The figure shows three views and two pictorial views of one solid part (mm, origin at its lowest corner). Answer the questions. A direction names the side the tool comes from. Coordinates: 2 decimals unless noted, no trailing zeros. Loops run counter-clockwise (first coordinate to the right, second up) from the corner with the lowest first, then second, coordinate; pieces in that order, holes last. Notation, with made-up numbers: M 85,-1 L 101,-1 A30 ccw 101,28 Z; hole C 82.5,75.25 d1. An arc over 180 degrees is marked long. Answer as a JSON object with one key per item and string values. Group by question number.
1. Straight lines are drawn through the part: L1, parallel to Y at x = 2.75, z = 2.25; L2, parallel to Z at x = 4, y = 11; L3, parallel to X at y = 5.5, z = 3. For each, find the intervals that lie inside material, in ascending order.
2. A cutting plane is placed at C-C on y = 12.75. Give the vertices of the cut face in (x, z).
3. Given pin 1 (0.5 mm diameter, centred on x = 3.5, y = 15, fed in from +Z); pin 2 (2 mm diameter, centred on x = 3, z = 3.5, fed in from +Y); pin 3 (3 mm diameter, centred on x = 2.5, y = 14, fed in from +Z); pin 4 (1.5 mm diameter, centred on y = 9.5, z = 3.5, fed in from -X), each flat-ended and moving along its own axis, determine where each tip first touches the part or whether it passes through.
4. A cutting plane is placed at A-A on y = 15.25. Give the vertices of the cut face in (x, z) (1 decimal).
5. For the marked faces 4, 5 and 6, determine the directions among +Z, -Z, +X, -X, +Y, -Y from which every point of the face is accessible in a straight line to the end or side of a thin tool.
6. A cutting plane is placed at B-B on x = 3.1. Give the vertices of the cut face in (y, z).
7. Determine the mould class of the marked faces 1, 2 and 3 for opening direction Z: released by +Z, released by -Z, zero draft, split by the parting line, or undercut.
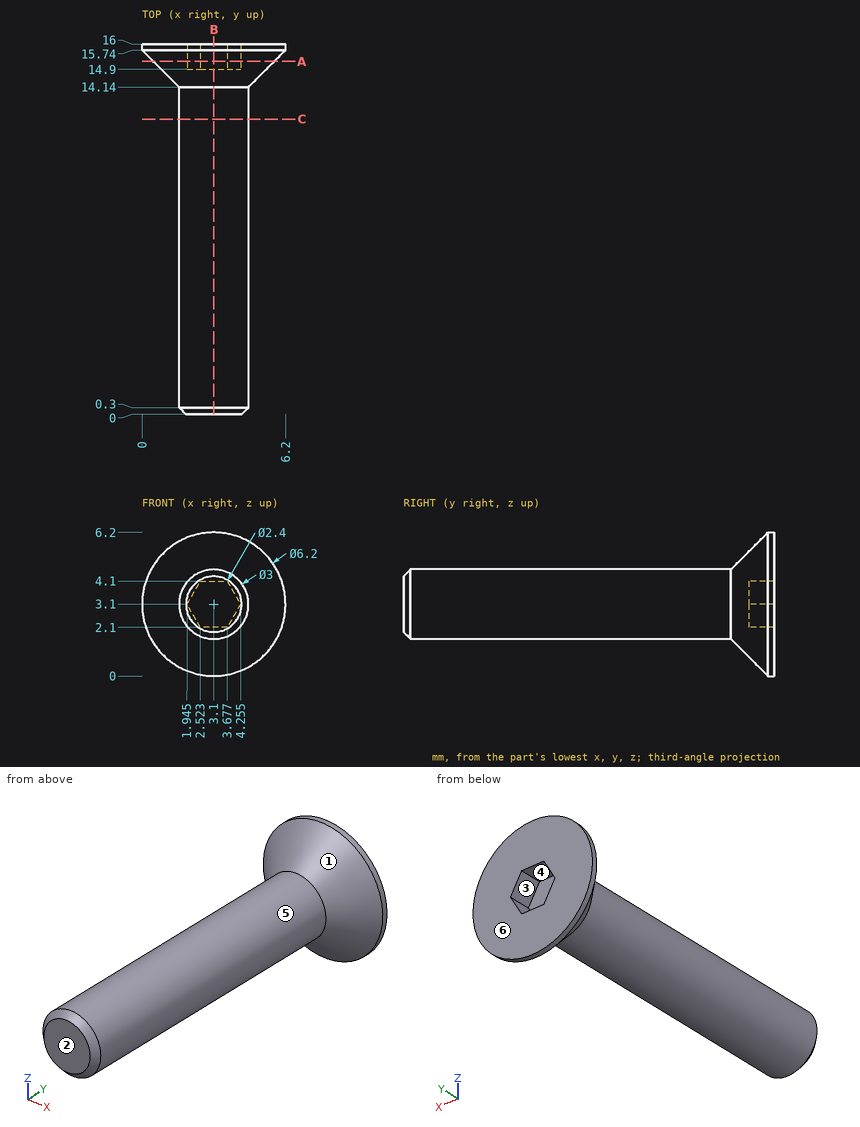
From the geometry:
{
 "1": {"L1": "y = 0 to 14.9", "L2": "z = 1.9 to 4.3", "L3": "x = 1.6 to 4.6"},
 "2": {"outline": "C 3.1,3.1 d3"},
 "3": {"pin 1": "stops at z = 5.68", "pin 2": "stops at y = 16", "pin 3": "stops at z = 5.92", "pin 4": "stops at x = 1.6"},
 "4": {"outline": "C 3.1,3.1 d5.2; hole M 1.9,3.1 L 2.5,2.1 L 3.7,2.1 L 4.3,3.1 L 3.7,4.1 L 2.5,4.1 Z"},
 "5": {"face 4": "+Y", "face 5": "-Y", "face 6": "+Z, -Z, +X, -X, +Y"},
 "6": {"outline": "M 0,1.9 L 0.3,1.6 L 14.14,1.6 L 15.74,0 L 16,0 L 16,2.1 L 14.9,2.1 L 14.9,4.1 L 16,4.1 L 16,6.2 L 15.74,6.2 L 14.14,4.6 L 0.3,4.6 L 0,4.3 Z"},
 "7": {"face 1": "split by the parting line", "face 2": "zero draft", "face 3": "undercut"}
}
